from build123d import *

# Parameters (mm, degrees)
F0_W     = 45
F0_H     = 45
F1_DEPTH = 510
F2_W     = 10
F2_H     = 60
F4_DEPTH = 30
F3_W     = 10
F3_H     = 60
F5_DEPTH = 30


with BuildPart() as f1:
    # F0 (on Top) → F1 (new body)
    with BuildSketch(Plane.XY):
        with Locations((-22.5, 22.5)):
            Rectangle(F0_W, F0_H)
    extrude(amount=F1_DEPTH)

    # F2 (on face) → F4 (cut)
    with BuildSketch(Plane.YZ):
        with Locations((22.5, 470)):
            Rectangle(F2_W, F2_H)
    extrude(amount=-F4_DEPTH, mode=Mode.SUBTRACT)

    # F3 (on face) → F5 (cut)
    with BuildSketch(Plane.XZ):
        with Locations((-22.5, 470)):
            Rectangle(F3_W, F3_H)
    extrude(amount=-F5_DEPTH, mode=Mode.SUBTRACT)


solid = f1.part
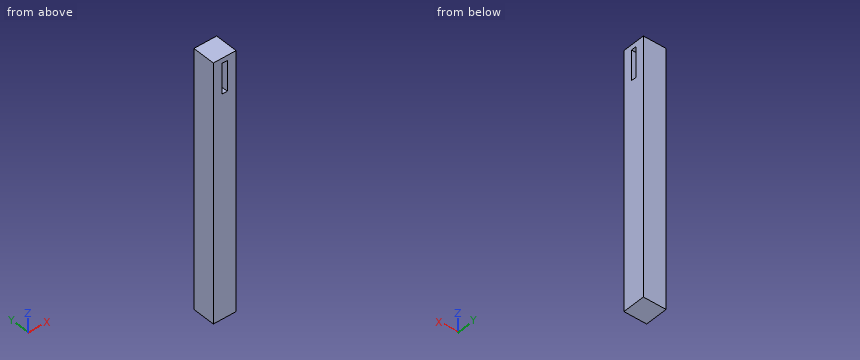
Input: part model. Units: mm. Frame: model coordinates. Coordinates: 2 decimals unless noted, no trailing zeros. Loops run counter-clockwise (first coordinate to the right, second up) from the corner with the lowest first, then second, coordinate; pieces in that order, holes last. Notation, with made-up numbers: (-20.75, 74.5) -> (29.25, 74.5) arc R21 cw to (29.25, 109.5) -> close; hole circle Ø3 at (72, 31.25). An arc over 180 degrees is marked (long way). Write each question's results on one line, items separated by ' | '. Start each with the question number.
Q1. Section A-A, the plane z = 476.5. Return the cut outline in (x, y), plus the area to 4 significant figures.
Q2. Ray query, line 1 (Y direction, x = -14, z = 454); line 2 (Z direction, x = -6, y = 23). Return the intervals inside material, ascending. Write a range as from..to.
Q3. Section B-B, the plane y = 5. Return the cut outline in (x, z), plus the area to 4 significant figures.
Q4. Pin query (flat end, axial travel): pin 1 (19 mm diameter, centred on y = 5.5, z = 478.5, fed in from +X); pin 2 (8 mm diameter, centred on x = -22, z = 474.5, fed in from -Y); pin 3 (5 mm diameter, centred on y = 24, z = 471.5, fed in from +X). Return the tip coordinate at first contact, or that it passes through.
Found:
1) outline: (-45, 0) -> (-27.5, 0) -> (-27.5, 17.5) -> (-30, 17.5) -> (-30, 27.5) -> (-27.5, 27.5) -> (-27.5, 30) -> (-17.5, 30) -> (-17.5, 27.5) -> (0, 27.5) -> (0, 45) -> (-45, 45) -> close; (-17.5, 0) -> (0, 0) -> (0, 17.5) -> (-17.5, 17.5) -> close | area: 1,525 mm2
2) line 1: 0..17.5, 27.5..45 | line 2: 0..440, 500..510
3) outline: (-45, 0) -> (0, 0) -> (0, 510) -> (-45, 510) -> close; hole (-27.5, 440) -> (-17.5, 440) -> (-17.5, 500) -> (-27.5, 500) -> close | area: 22,350 mm2
4) pin 1: x = 0 | pin 2: y = 30 | pin 3: x = -30
